Drawing for the job (mm, zero at the part's lowest x, y, z). Give positions to 0.01 mm unless a question says otherwise; leave off trailing zeros. Loops run counter-clockwise (first coordinate to the right, second up) from the corner with the lowest first, then second, coordinate; pieces in that order, holes last.
1) Wall check: line 1 (Y direction, x = 3, z = 0.65); line 2 (X direction, y = 3, z = 0.2). Give the ranges that are in metal, low to high.
2) Band-saw the part on B-B on z = 0.3. List the corners of the cut face in (x, y), then the cut area to 3 significant figures.
3) Two-plate mould, pull along Z, no slides. Class the marked faces 1 and 2: +Z half, -Z half, draft (parallel to the pull), parting line (faces both ways), or undercut.
4) Band-saw the part on A-A on y = 20. List the corners of the cut face in (x, z), then the cut area to 3 significant figures.
5) Flat gauge pin, fed straight in: P1, Ø3.5, axis at x = 37, y = 20, coming from the +Z side. Where does the tip first touch, or does it go through?
6) Band-saw the part on C-C on x = 36. List the corners of the cut face in (y, z), then the cut area to 3 significant figures.
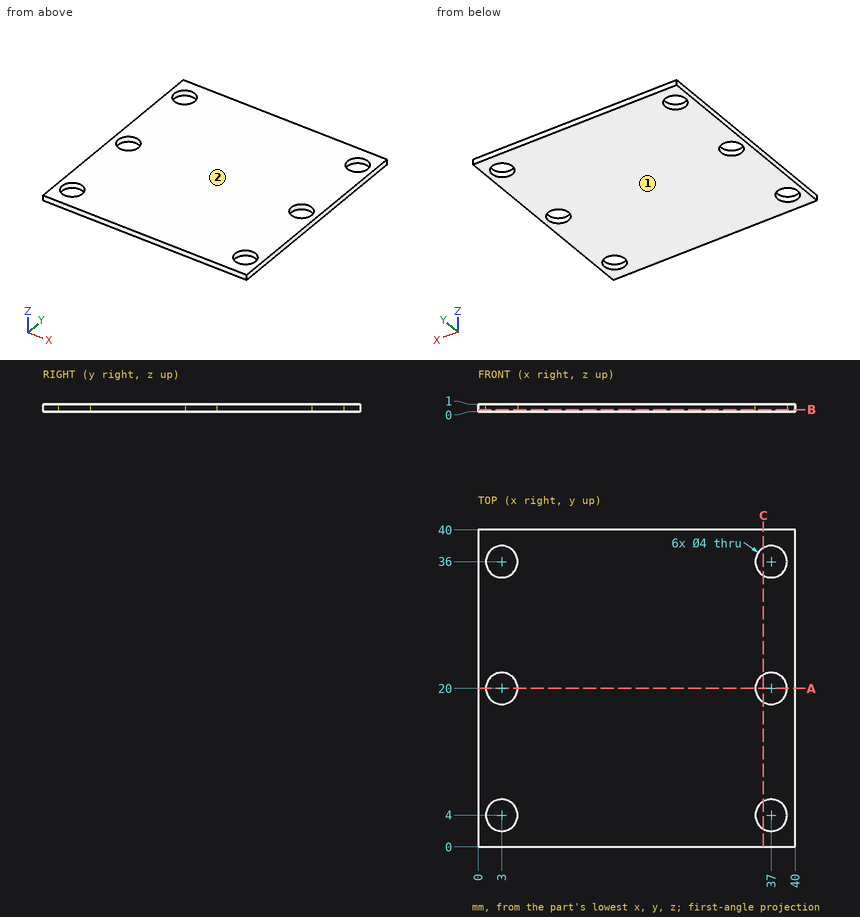
Findings below:
1. line 1: y = 0 to 2, 6 to 18, 22 to 34, 38 to 40
1. line 2: x = 0 to 1.27, 4.73 to 35.27, 38.73 to 40
2. outline: (0, 0) - (40, 0) - (40, 40) - (0, 40) - close; hole circle Ø4 at (3, 4); hole circle Ø4 at (3, 20); hole circle Ø4 at (3, 36); hole circle Ø4 at (37, 4); hole circle Ø4 at (37, 20); hole circle Ø4 at (37, 36)
2. area: 1,520 mm2
3. face 1: -Z half
3. face 2: +Z half
4. outline: (0, 0) - (1, 0) - (1, 1) - (0, 1) - close; (5, 0) - (35, 0) - (35, 1) - (5, 1) - close; (39, 0) - (40, 0) - (40, 1) - (39, 1) - close
4. area: 32.0 mm2
5. P1: passes through
6. outline: (0, 0) - (2.27, 0) - (2.27, 1) - (0, 1) - close; (5.73, 0) - (18.27, 0) - (18.27, 1) - (5.73, 1) - close; (21.73, 0) - (34.27, 0) - (34.27, 1) - (21.73, 1) - close; (37.73, 0) - (40, 0) - (40, 1) - (37.73, 1) - close
6. area: 29.6 mm2
